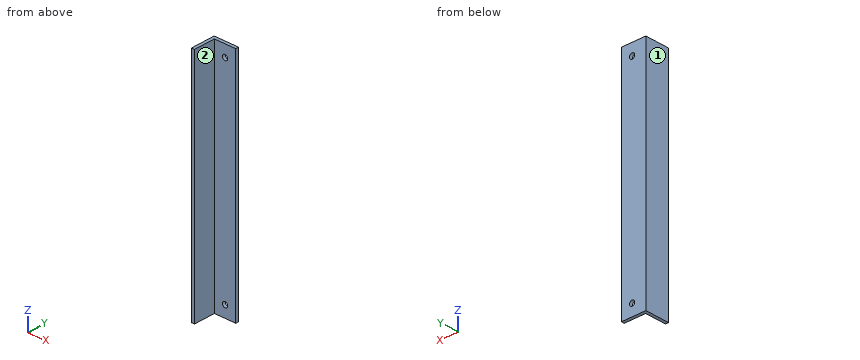
Autodesk Fusion 360 part; units mm, degrees
sketch "Sketch1" plane through (0, 0, 0) normal (0, 0, 1) x (1, 0, 0)
  line L0 (0, 0) -> (25.4, 0)
  line L1 (0, 0) -> (0, -25.4)
  line L2 (3.175, -3.175) -> (25.4, -3.175)
  line L3 (3.175, -3.175) -> (3.175, -25.4)
  line L4 (25.4, 0) -> (25.4, -3.175)
  line L5 (0, -25.4) -> (3.175, -25.4)
  dimension "d1" = 25.4
  dimension "d2" = -3.175
extrude "Extrude1" add sketch "Sketch1" along normal blind 240
sketch "Sketch2" plane through (0, -3.175, 0) normal (0, -1, 0) x (1, 0, 0)
  line L0 (3.175, 0) -> (25.4, 0)
  line L1 (25.4, 0) -> (25.4, 240)
  line L2 (25.4, 240) -> (3.175, 240)
  line L3 (3.175, 240) -> (3.175, 0)
  circle A0 centre (14.2875, 228) radius 2.75
  circle A1 centre (14.2875, 12) radius 2.75
  line L4 (14.2875, 240) -> (14.2875, 0) construction
  dimension "d5" = 5.5
  dimension "d6" = 12
  dimension "d7" = 12
hole "Hole1" at (14.2875, -3.175, 12) at (14.2875, -3.175, 228) direction (0, 1, 0) diameter 5.5 depth 7 tip angle 118
CAD build for the part. Positions are in the model's coordinates, mm. Face numbers are marked on the shaded views. A direction names the side the tool comes from. Coordinates: 2 decimals unless noted, no trailing zeros. Write each loop counter-clockwise with the first axis right and the second up, starting at its lowest first coordinate (ties: lowest second). Pieces come first, ordered by that corner, then holes. Notation, with made-up numbers: (19, 68.5) - (59, 68.5) arc R11 cw to (59, 89.5) - close; hole circle Ø2 at (63, -2). An arc over 180 degrees is marked (long way). Use a Markdown table: item, result. Add a question column.
Item 1: Band-saw the part on A-A, the plane z = 228. Give the cut face in (x, y) (1 decimal).
Item 2: 3-axis set-ups, long thin cutter, end or side, ignore diameter. For the marked faces 1 and 2: which of +Z, -Z, +X, -X, +Y, -Y reach the whole face in a straight line?
Item 3: Flat gauge pins, fed straight in: pin 1 (6.5 mm diameter, centred on x = 15, z = 127.5, fed in from -Y) (3 decimals); pin 2 (12 mm diameter, centred on y = -11.5, z = 169.5, fed in from +X) (3 decimals). Where does each tip first touch, or does it go through?
Item 4: Band-saw the part on B-B, the plane z = 204. Give the cut face in (x, y) (3 decimals), and give its area (3 significant figures).
Item 5: Band-saw the part on C-C, the plane y = -13.5. Give the cut face in (x, z) (3 decimals), and give its area (3 significant figures).
Item 6: Drill centre lines: L1, parallel to X at y = -1.45, z = 12; L2, parallel to Y at x = 16.75, z = 170 (3 decimals); L3, parallel to X at y = -9, z = 160 (3 decimals). Where is each one in solid material? Low to high. Write a range as from..to.
Numbers:
| question | item | result |
|---|---|---|
| 1 | outline | (0, -25.4) - (3.2, -25.4) - (3.2, -3.2) - (11.5, -3.2) - (11.5, 0) - (0, 0) - close; (17, -3.2) - (25.4, -3.2) - (25.4, 0) - (17, 0) - close |
| 2 | face 1 | +Z, -Z, -X, +Y, -Y |
| 2 | face 2 | +Z, -Z, +X, -Y |
| 3 | pin 1 | y = -3.175 |
| 3 | pin 2 | x = 3.175 |
| 4 | outline | (0, -25.4) - (3.175, -25.4) - (3.175, -3.175) - (25.4, -3.175) - (25.4, 0) - (0, 0) - close |
| 4 | area | 151 mm2 |
| 5 | outline | (0, 0) - (3.175, 0) - (3.175, 240) - (0, 240) - close |
| 5 | area | 762 mm2 |
| 6 | L1 | 0..11.54, 17.04..25.4 |
| 6 | L2 | -3.175..0 |
| 6 | L3 | 0..3.175 |
